```python
from build123d import *

# Parameters (mm, degrees)
F1_DEPTH = 25.4
F2_DEPTH = 2.54


with BuildPart() as f1:
    # F0 (on Front) → F1 (new body)
    with BuildSketch(Plane.XZ):
        Polygon((-120.65, 139.7), (120.65, 139.7), (120.65, -139.7), (120.65, -140.171826), (123.63416, -140.171826), (123.63416, 140.171826), (-123.63416, 140.171826), (-123.63416, -140.171826), (-120.65, -140.171826), (-120.65, -139.7), align=None)
    extrude(amount=F1_DEPTH)

    # F0 (on Front) → F2 (join)
    with BuildSketch(Plane.XZ):
        Polygon((120.65, -139.7), (120.65, 139.7), (-120.65, 139.7), (-120.65, -139.7), (-120.65, -140.171826), (120.65, -140.171826), align=None)
    extrude(amount=F2_DEPTH)


solid = f1.part
```
The model under review builds one solid part; all positions refer to its coordinate system, in mm. A direction names the side the tool comes from. Round coordinates to 2 decimals unless told otherwise and drop trailing zeros. Order: outer loops, then holes, each group sorted by start corner. A loop starts at its lowest first (then second) coordinate and runs counter-clockwise, first axis right, second up. Notation, with made-up numbers: M 79,28 L 138,28 A23 cw 138,43 Z; hole C -31.5,16.5 d2. An arc over 180 degrees is marked long. Use a Markdown table: item, result.
1) Consider section B-B (y = -7.25). Write out the cut boundary in (x, z), then the cut area to 3 significant figures.
Report:
| item | result |
|---|---|
| outline | M -123.63,-140.17 L -120.65,-140.17 L -120.65,139.7 L 120.65,139.7 L 120.65,-140.17 L 123.63,-140.17 L 123.63,140.17 L -123.63,140.17 Z |
| area | 1,790 mm^2 |
2) Insertion check: pin 1 (8 mm diameter, centred on x = -5.5, y = -10, fed in from -Z); pin 2 (4 mm diameter, centred on x = -9.5, z = -6.5, fed in from -Y). Each pin has a flat end and moves straight along its axis. Give the tip position at first contact, or say it passes through.
Report:
| item | result |
|---|---|
| pin 1 | z = 139.7 |
| pin 2 | y = -2.54 |
3) Wall thickness on line 1 along X through (y, z) = (-3.5, 37); line 2 along Y through (x, z) = (50, -98); line 3 along Z through (x, y) = (-67.5, -19.5): over which ranges is each line inside the solid? List them lowest first. Write a range as [from, to].
Report:
| item | result |
|---|---|
| line 1 | [-123.63, -120.65], [120.65, 123.63] |
| line 2 | [-2.54, 0] |
| line 3 | [139.7, 140.17] |
4) Tool access review of faces 4 (the face through (-123.634, -13, 2)), 5 (the face through (-120.65, -14, -2)): name each direction out of +Z, -Z, +X, -X, +Y, -Y from which nothing blocks a thin tool from reaching the whole face with its end or side.
Report:
| item | result |
|---|---|
| face 4 | +Z, -Z, -X, +Y, -Y |
| face 5 | -Z, -Y |
5) Consider section A-A (z = 15). Write out the cut boundary in (x, y), then the cut area to 3 significant figures.
Report:
| item | result |
|---|---|
| outline | M -123.63,-25.4 L -120.65,-25.4 L -120.65,-2.54 L 120.65,-2.54 L 120.65,-25.4 L 123.63,-25.4 L 123.63,0 L -123.63,0 Z |
| area | 764 mm^2 |
6) Consider section C-C (x = -76.5). Write out the cut boundary in (y, z).
Report:
| item | result |
|---|---|
| outline | M -25.4,139.7 L -2.54,139.7 L -2.54,-140.17 L 0,-140.17 L 0,140.17 L -25.4,140.17 Z |
7) Draft analysis for pull direction X (two halves, no side actions). For faces 1 (the face through (123.634, -13, -2)), 2 (the face through (120.65, -14, 2)), 3 (the face through (2, -13, 140.172)), state which applies: released by +X, released by -X, zero draft, split by the parting line, or undercut.
Report:
| item | result |
|---|---|
| face 1 | released by +X |
| face 2 | undercut |
| face 3 | zero draft |
